```python
from build123d import *

# Parameters (mm, degrees)
F0_W     = 60
F0_H     = 100
F0_R     = 3
F0_R_2   = 2
F0_R_3   = 4
F1_DEPTH = 5
F3_DEPTH = 55
F5_DEPTH = 75.001
F6_R     = 15
F6_R_2   = 2
F7_DEPTH = 25.001


with BuildPart() as f1:
    # F0 (on Top) → F1 (new body)
    with BuildSketch(Plane.XY):
        with Locations((30, 50)):
            Rectangle(F0_W, F0_H)
        with Locations((10, 10)):
            Circle(F0_R, mode=Mode.SUBTRACT)
        with Locations((50, 10)):
            Circle(F0_R, mode=Mode.SUBTRACT)
        with Locations((10, 55)):
            Circle(F0_R_2, mode=Mode.SUBTRACT)
        with Locations((50, 55)):
            Circle(F0_R_2, mode=Mode.SUBTRACT)
        with Locations((30, 90)):
            Circle(F0_R_3, mode=Mode.SUBTRACT)
    extrude(amount=F1_DEPTH)

    # F2 (on face) → F3 (join)
    with BuildSketch(Plane.XY.offset(5)):
        Polygon((25, 74), (5, 74), (5, 71), (22, 71), (22, 28), (5, 28), (5, 25), (25, 25), align=None)
    extrude(amount=F3_DEPTH)

    # F4 (on face) → F5 (cut, through all)
    with BuildSketch(Plane.XZ.offset(-25)):
        Polygon((22, 60), (5, 60), (5, 10), align=None)
    extrude(amount=-F5_DEPTH, mode=Mode.SUBTRACT)

    # F6 (on face) → F7 (cut, through all)
    with BuildSketch(Plane.YZ.offset(25)):
        with Locations((49.5, 39)):
            Circle(F6_R)
        with Locations((34, 54.5)):
            Circle(F6_R_2)
        with Locations((65, 54.5)):
            Circle(F6_R_2)
        with Locations((65, 23.5)):
            Circle(F6_R_2)
        with Locations((34, 23.5)):
            Circle(F6_R_2)
    extrude(amount=-F7_DEPTH, mode=Mode.SUBTRACT)


solid = f1.part
```
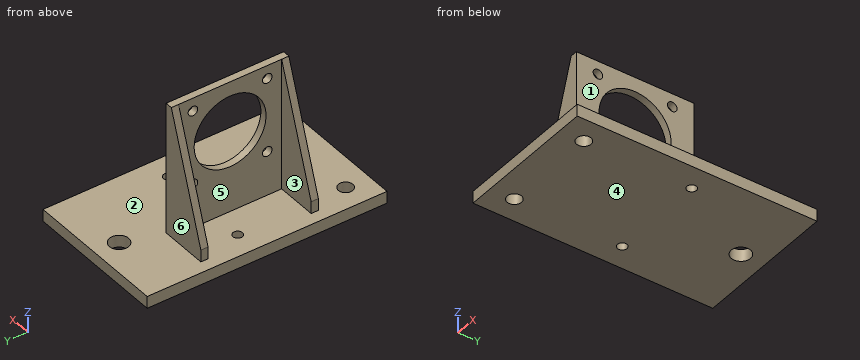
The listing builds one solid part. Answer for the finished solid, in the listing's coordinates (mm). Face numbers are marked on the shaded views. A direction names the side the tool comes from. Give positions to 0.01 mm unless a question says otherwise; leave off trailing zeros. Order: outer loops, then holes, each group sorted by start corner. A loop starts at its lowest first (then second) coordinate and runs counter-clockwise, first axis right, second up. Notation, with made-up numbers: M 51.25,80 L 71.25,80 A22 ccw 71.25,95 Z; hole C 31.5,34.5 d5. An arc over 180 degrees is marked long. Put each result on its own line as item: value. Start each with the question number.
Item 1: For a pull along Y with two mould halves and no side action, classify the marked faces 3, 4, 5 and 6 as +Y half, -Y half, draft (parallel to the pull), parting line (faces both ways), or undercut.
Item 2: The part is cut by section C-C, the plane z = 8. Determine the outline of the cut face in (x, y), and give its area (3 significant figures).
Item 3: Find the intervals of material crossed by line 1 along Y through (x, z) = (10, 1); line 2 along Z through (x, y) = (23.2, 34); line 3 along Y through (x, z) = (30, 1), in increasing order.
Item 4: The part is cut by section A-A, the plane z = 39. Determine the outline of the cut face in (x, y).
Item 5: Flat-ended cylindrical pins translate along their axes: P1, Ø12, axis at x = 21, z = 11.5, coming from the -Y side; P2, Ø3.5, axis at y = 26, z = 8, coming from the -X side; P3, Ø4, axis at x = 14, y = 78, coming from the +Z side. Find the tip coordinate at first contact, or state that the pin passes through.
Item 6: Which of the six approach directions +Z, -Z, +X, -X, +Y, -Y give full straight-line access (tool end or side, diameter ignored) to the marked faces 1 and 2?
Item 7: The part is cut by section D-D, the plane x = 16. Determine the outline of the cut face in (y, z).
Item 8: The part is cut by section B-B, the plane y = 49.5. Determine the outline of the cut face in (x, z), and give its area (3 significant figures).
Answer key:
1. face 3: undercut
1. face 4: draft
1. face 5: undercut
1. face 6: +Y half
2. outline: M 5,25 L 25,25 L 25,74 L 5,74 L 5,71 L 22,71 L 22,28 L 5,28 Z
2. area: 249 mm²
3. line 1: y = 0 to 7, 13 to 53, 57 to 100
3. line 2: z = 0 to 21.5, 25.5 to 52.5, 56.5 to 60
3. line 3: y = 0 to 86, 94 to 100
4. outline: M 14.86,25 L 25,25 L 25,34.5 L 22,34.5 L 22,28 L 14.86,28 Z; M 14.86,71 L 22,71 L 22,64.5 L 25,64.5 L 25,74 L 14.86,74 Z
5. P1: stops at y = 25
5. P2: stops at x = 5
5. P3: stops at z = 5
6. face 1: +Z, +X, +Y, -Y
6. face 2: +Z
7. outline: M 0,0 L 100,0 L 100,5 L 74,5 L 74,42.35 L 71,42.35 L 71,5 L 28,5 L 28,42.35 L 25,42.35 L 25,5 L 0,5 Z
8. outline: M 0,0 L 60,0 L 60,5 L 25,5 L 25,24 L 22,24 L 22,5 L 0,5 Z; M 22,54 L 25,54 L 25,60 L 22,60 Z
8. area: 375 mm²
